```python
from build123d import *

# Parameters (mm, degrees)
SZKIC3_R                    = 47.5
SZKIC3_R_2                  = 6.25
DODANIE_WYCI_GNI_CIE2_DEPTH = 10


with BuildPart() as part:
    # Szkic3 → Dodanie-wyciągnięcie2 (new body)
    with BuildSketch(Plane(origin=(0, 0, 0), x_dir=(1, 0, 0), z_dir=(0, 1, 0))):
        Polygon((-77.5, 77.5), (77.5, 77.5), (77.5, -77.5), (77.5, -92.5), (-109.948637287, -92.5), (-155.5, 77.5), align=None)
        Circle(SZKIC3_R, mode=Mode.SUBTRACT)
        with Locations((62.5, 62.5)):
            Circle(SZKIC3_R_2, mode=Mode.SUBTRACT)
        with Locations((62.5, -57.5)):
            Circle(SZKIC3_R_2, mode=Mode.SUBTRACT)
        with Locations((-88.268573609, -57.5)):
            Circle(SZKIC3_R_2, mode=Mode.SUBTRACT)
        with Locations((-108.974097218, 19.774066103)):
            Circle(SZKIC3_R_2, mode=Mode.SUBTRACT)
    extrude(amount=DODANIE_WYCI_GNI_CIE2_DEPTH)


solid = part.part
```
CAD build for the part. Positions are in the model's coordinates, mm. Round coordinates to 2 decimals unless told otherwise and drop trailing zeros. Write each loop counter-clockwise with the first axis right and the second up, starting at its lowest first coordinate (ties: lowest second). Pieces come first, ordered by that corner, then holes. Notation, with made-up numbers: M 15.25,71.5 L 54.25,71.5 A16 cw 54.25,100.5 Z; hole C -20.5,49.25 d6. An arc over 180 degrees is marked long. One line per question, with ' | ' between items.
1. Cut at D-D on z = 0. Write the cut outline in (x, y).
Working result:
outline: M -134.73,0 L -47.5,0 L -47.5,10 L -134.73,10 Z; M 47.5,0 L 77.5,0 L 77.5,10 L 47.5,10 Z
2. Cut at B-B on z = 57.5. Write the cut outline in (x, y).
Working result:
outline: M -119.33,0 L -94.52,0 L -94.52,10 L -119.33,10 Z; M -82.02,0 L 56.25,0 L 56.25,10 L -82.02,10 Z; M 68.75,0 L 77.5,0 L 77.5,10 L 68.75,10 Z
3. Probe L1, parallel to Z at x = 62.5, y = 5.25; L2, parallel to Z at x = 1.5, y = 4; L3, parallel to X at y = 8.75, z = -20. List the from-to ranges inside material, lowest first. Write a range as from..to.
Working result:
L1: -77.5..-68.75, -56.25..51.25, 63.75..92.5 | L2: -77.5..-47.48, 47.48..92.5 | L3: -140.09..-115.22, -102.73..-43.08, 43.08..77.5
4. Cut at A-A on x = 0. Write the cut outline in (y, z).
Working result:
outline: M 0,-77.5 L 10,-77.5 L 10,-47.5 L 0,-47.5 Z; M 0,47.5 L 10,47.5 L 10,92.5 L 0,92.5 Z
5. Cut at C-C on x = 62.5. Write the cut outline in (y, z).
Working result:
outline: M 0,-77.5 L 10,-77.5 L 10,-68.75 L 0,-68.75 Z; M 0,-56.25 L 10,-56.25 L 10,51.25 L 0,51.25 Z; M 0,63.75 L 10,63.75 L 10,92.5 L 0,92.5 Z
6. Mould opens along X. For faces 1 (the flat face through (77.5, 5, 9)), 2 (the cylindrical face through (-103.013, 4.93, -21.651)), 3 (the flat face through (-63, 0, 6)) say: pulls with the +X half, pulls with the -X half, needs draft (parallel to the pull), parting line crosses it, or undercut.
Working result:
face 1: pulls with the +X half | face 2: undercut | face 3: needs draft
7. Pin check, flat tip, straight feed: pin 1 Ø1 at (x, z) = (51, 19) entering from -Y. Stop position of the tip, or through.
Working result:
pin 1: y = 0
